Autodesk Inventor part; units mm, degrees
ref_plane "YZ Plane" through (0, 0, 0) normal (1, 0, 0) x (0, 1, 0)
ref_plane "XZ Plane" through (0, 0, 0) normal (0, 1, 0) x (-1, 0, 0)
ref_plane "XY Plane" through (0, 0, 0) normal (0, 0, 1) x (1, 0, 0)
sketch "Sketch1" plane through (0, 0, 0) normal (0, 0, 1) x (1, 0, 0)
  line L0 (0, 0) -> (101.6, 0)
  line L1 (101.6, 0) -> (101.6, 373.888)
  line L2 (101.6, 373.888) -> (0, 373.888)
  line L3 (0, 373.888) -> (0, 0)
  dimension "d0" = 101.6
  dimension "d1" = 373.888
extrude "Extrusion1" add sketch "Sketch1" against normal blind 6.35
sketch "Sketch2" plane through (0, 0, 0) normal (0, 0, 1) x (1, 0, 0)
  line L0 (101.6, 0) -> (101.6, 373.888)
  line L1 (50.3784, 186.944) -> (-65.1556, 186.944) construction
  line L2 (0, 228.5746) -> (-60.1541, 228.5746) construction
  line L3 (101.6, 279.3746) -> (139.7, 279.3746)
  line L4 (139.7, 279.3746) -> (139.7, 177.7746)
  line L5 (139.7, 177.7746) -> (101.6, 177.7746)
  line L6 (101.6, 177.7746) -> (101.6, 279.3746)
  line L7 (0, 0) -> (101.6, 0) construction
  line L8 (101.6, 373.888) -> (0, 373.888) construction
  point P0 (101.6, 228.5746)
  dimension "d50" = 41.6306
  dimension "d51" = 38.1
  dimension "d52" = 101.6
  dimension "d53" = 373.888
  dimension "d54" = 186.944
extrude "Extrusion2" add sketch "Sketch2" against normal blind 6.35
fillet "Fillet1" radius 3.175 1 edges at (101.6, 279.3746, -3.175)
fillet "Fillet2" radius 3.175 1 edges at (101.6, 177.7746, -3.175)
sketch "Sketch3" plane through (0, 0, 0) normal (0, 0, 1) x (1, 0, 0)
  line L0 (101.6, 0) -> (101.6, 174.5996)
  line L1 (0, 0) -> (101.6, 0)
  point P0 (44.45, 7.62)
  point P1 (101.6, 132.969)
  point P2 (101.6, 180.594)
  dimension "d11" = 57.15
  dimension "d12" = 7.62
hole "Hole1" at (44.45, 7.62, 0) direction (0, 0, -1) diameter 5.08 end through all
ref_plane "Work Plane1" through (50.8, 0, 0) normal (-1, 0, 0) x (0, 0, 1)
pattern_linear "Rectangular Pattern1" count 2 spacing 12.7 along (1, 0, 0) count 5 spacing 89.662 along (0, 1, 0) of "Hole1"
ref_plane "Work Plane4" through (139.7, 228.5746, -6.35) normal (0, -1, 0) x (1, 0, 0)
sketch "Sketch6" plane through (0, 0, 0) normal (0, 0, 1) x (1, 0, 0)
  line L0 (139.7, 279.3746) -> (139.7, 177.7746) construction
  line L1 (139.7, 177.7746) -> (104.775, 177.7746) construction
  point P0 (0, 0)
  point P1 (114.3, 185.3946)
  dimension "d56" = 25.4
  dimension "d57" = 7.62
hole "Hole4" at (114.3, 185.3946, 0) direction (0, 0, -1) diameter 5.08 end through all
mirror "Mirror3" about plane through (139.7, 228.5746, -6.35) normal (0, -1, 0) of "Hole4"
sketch "Sketch7" plane through (0, 0, 0) normal (0, 0, 1) x (1, 0, 0)
  line L0 (0, 373.888) -> (0, 0) construction
  line L1 (167.64, 228.5746) -> (-27.94, 228.5746)
  point P0 (86.2584, 241.2746)
  dimension "d65" = 86.2584
  dimension "d73" = 12.7
hole "Hole5" at (86.2584, 241.2746, 0) direction (0, 0, -1) diameter 5.08 end through all
pattern_linear "Rectangular Pattern3" count 2 spacing 25.4 along (0, -1, 0) count 2 spacing 44.45 along (1, 0, 0) of "Hole5"
properties part number "Backhoe to Frame Mount"
The listing builds one solid part. Answer for the finished solid, in the listing's coordinates (mm). A direction names the side the tool comes from. Coordinates: 2 decimals unless noted, no trailing zeros. Write each loop counter-clockwise with the first axis right and the second up, starting at its lowest first coordinate (ties: lowest second). Pieces come first, ordered by that corner, then holes. Notation, with made-up numbers: (10.25, 35) - (49.25, 35) arc R9 cw to (49.25, 39) - close; hole circle Ø3 at (44, -11). An arc over 180 degrees is marked (long way). Return JSON: item names as keys, results as strings.
1. Which of the six approach directions +Z, -Z, +X, -X, +Y, -Y give full straight-line access (tool end or side, diameter ignored) to faces 1 (the face through (53, 190, -6.35)), 2 (the face through (101.6, 86, -3)), 3 (the face through (101.6, 328, -3))?
Final values:
{"face 1": "-Z, +X, -X, +Y, -Y", "face 2": "+Z, -Z, +X, -Y", "face 3": "+Z, -Z, +X, +Y"}
2. The part is cut by section B-B on y = 286. Determine the outline of the cut face in (x, z), then the cut area to 3 significant figures.
Final values:
{"outline": "(0, -6.35) - (101.6, -6.35) - (101.6, 0) - (0, 0) - close", "area": "645 mm^2"}
3. Each of these flat-tipped pins is pushed along its axis until it touches: pin 1 Ø3 at (y, z) = (310.5, -3) entering from +X; pin 2 Ø1.5 at (x, z) = (100.5, -4.5) entering from -Y. Where does it stop, or does it pass through?
Final values:
{"pin 1": "x = 101.6", "pin 2": "y = 0"}
4. The part is cut by section A-A on z = -3.5. Count the separate pieces of the cut face and the enclosed holes in it, then the cut area to 3 significant figures.
Final values:
{"separate pieces": "1", "enclosed holes": "16", "area": "41,500 mm^2"}
5. Consider line 1 along X through (y, z) = (7.62, -2); line 2 along Y through (x, z) = (114.3, -1.5); line 3 along Y through (x, z) = (44.45, -3.5). Determine where each line is inside the solid, lowest interval first.
Final values:
{"line 1": "0 to 41.91, 46.99 to 54.61, 59.69 to 101.6", "line 2": "177.77 to 182.85, 187.93 to 269.21, 274.29 to 279.37", "line 3": "0 to 5.08, 10.16 to 94.74, 99.82 to 184.4, 189.48 to 274.07, 279.15 to 363.73, 368.81 to 373.89"}
